Model file for the job. Use its own axes, mm. Coordinates: 2 decimals unless noted, no trailing zeros. Loops run counter-clockwise (first coordinate to the right, second up) from the corner with the lowest first, then second, coordinate; pieces in that order, holes last. Notation, with made-up numbers: (35, -14.5) -> (92, -14.5) arc R29 cw to (92, 18.5) -> close; hole circle Ø10 at (7.5, 45). An arc over 180 degrees is marked (long way). Use one line per item in the form item = value.
Autodesk Inventor part; units mm, degrees
ref_plane "YZ Plane" through (0, 0, 0) normal (1, 0, 0) x (0, 1, 0)
ref_plane "XZ Plane" through (0, 0, 0) normal (0, 1, 0) x (-1, 0, 0)
ref_plane "XY Plane" through (0, 0, 0) normal (0, 0, 1) x (1, 0, 0)
sketch "Sketch1" plane through (0, 0, 0) normal (0, 0, 1) x (1, 0, 0)
  circle A0 centre (0, 0) radius 1.3341
  dimension "d0" = 2.6682
extrude "Extrusion1" add sketch "Sketch1" along normal mid plane 7.137
sketch "Sketch2" plane through (0, 0, 3.5685) normal (0, 0, 1) x (1, 0, 0)
  circle A0 centre (0, 0) radius 0.25
  dimension "d7" = 0.5
sketch3d "3D Sketch2"
sweep "Sweep1" [suppressed]
sketch "Sketch3" plane through (0, 0, -3.5685) normal (0, 0, -1) x (-1, 0, 0)
  circle A0 centre (0, 0) radius 0.25
  dimension "d18" = 0.5
sketch3d "3D Sketch3"
sweep "Sweep2" [suppressed]
sketch "Sketch4" plane through (0, 0, 3.5685) normal (0, 0, 1) x (1, 0, 0)
  circle A0 centre (0, 0) radius 0.25
  dimension "d25" = 0.5
sketch3d "3D Sketch4"
sweep "Sweep3" [suppressed]
sketch "Sketch5" plane through (0, 0, -3.5685) normal (0, 0, -1) x (-1, 0, 0)
  circle A0 centre (0, 0) radius 0.254
  dimension "d34" = 0.508
sketch3d "3D Sketch5"
  line L0 (0, 0, -3.5685) -> (0, 0, -5.0685)
  arc A0 (0, 0, -5.0685) -> (-2, 0, -7.0685) centre (-2, 0, -5.0685) ccw
  line L1 (-2, 0, -7.0685) -> (-4, 0, -7.0685)
  dimension "d52" = 3.5
  dimension "d53" = 4
  dimension "d36" = 2
sweep "Sweep4" add profiles "Sketch5" path "3D Sketch5"
sketch "Sketch7" plane through (0, 0, 3.5685) normal (0, 0, 1) x (1, 0, 0)
  circle A0 centre (0, 0) radius 1.3341
  circle A1 centre (0, 0) radius 0.254
  dimension "d45" = 0.508
sketch3d "3D Sketch7"
sweep "Sweep6" [suppressed]
mirror "Mirror2" about plane through (0, 0, 0) normal (0, 0, 1) of "Sweep4"
properties part number "VISHAY-DALE RWR81S6R98FRB12" material "SMT (95% LCP, 5% PhosBr)"
Q1. Wall check: line 1 along X through (y, z) = (0.1, -1.5); line 2 along Z through (x, y) = (0.6, -0.2). Give the ranges that are in metal, low to high.
Result:
line_1 = -1.33 to 1.33
line_2 = -3.57 to 3.57
Q2. Band-saw the part on B-B, the plane y = -0.8. Write the cut outline in (x, z), and give its area (3 significant figures).
Result:
outline = (-1.07, -3.57) -> (1.07, -3.57) -> (1.07, 3.57) -> (-1.07, 3.57) -> close
area = 15.2 mm2
Q3. Pin check, flat tip, straight feed: pin 1 Ø1.3 at (x, y) = (0, 0.5) entering from +Z. Stop position of the tip, or through.
Result:
pin_1 = 6.74
Q4. Band-saw the part on A-A, the plane y = 0. Write the cut outline in (x, z), and give its area (3 significant figures).
Result:
outline = (-4, -7.32) -> (-2, -7.32) arc R2.25 ccw to (0.25, -5.07) -> (0.25, -3.57) -> (1.33, -3.57) -> (1.33, 3.57) -> (0.25, 3.57) -> (0.25, 5.07) arc R2.25 ccw to (-2, 7.32) -> (-4, 7.32) -> (-4, 6.81) -> (-2, 6.81) arc R1.75 cw to (-0.25, 5.07) -> (-0.25, 3.57) -> (-1.33, 3.57) -> (-1.33, -3.57) -> (-0.25, -3.57) -> (-0.25, -5.07) arc R1.75 cw to (-2, -6.81) -> (-4, -6.81) -> close
area = 25.8 mm2
